Can you work these out from the drawing? Everything is in mm from the part's minimum corner. A direction names the side the tool comes from. Give positions to 0.01 mm unless a question says otherwise; leave off trailing zeros. Order: outer loops, then holes, each group sorted by start corner. A loop starts at its lowest first (then second) coordinate and runs counter-clockwise, first axis right, second up. Notation, with made-up numbers: M 60.5,67 L 77.5,67 A21 cw 77.5,101 Z; hole C -21.5,80 d1. An arc over 180 degrees is marked long. Use a Markdown table: item, result. Add a question column.
Item 1: If I drill on L1, parallel to X at y = 9, z = 31; L2, parallel to X at y = 4, z = 8; L3, parallel to Y at x = 5, z = 28.5, over which ranges is the centre line in solid material (lowest first)? Write a range as from..to.
Item 2: For the marked faces 4 and 5, which set-ups out of +Z, -Z, +X, -X, +Y, -Y let a thin tool reach every point of the face, with its end or its side?
Item 3: If we mould it in two halves opening along X, with no side actions, what happens to the marked faces 1, 2 and 3? For each: released by +X, released by -X, zero draft, split by the parting line, or undercut.
Item 4: Suppose I cut it at A-A on z = 44.5. Write out the boundary of the cut face in (x, y).
Item 5: I'm going to push a flat-ended pin straight in: pin 1 Ø3.5 at (x, z) = (4.5, 47) entering from -Y. Where does the tip first touch, or does it pass through?
Item 6: Suppose I cut it at B-B on y = 2.25. Write out the boundary of the cut face in (x, z).
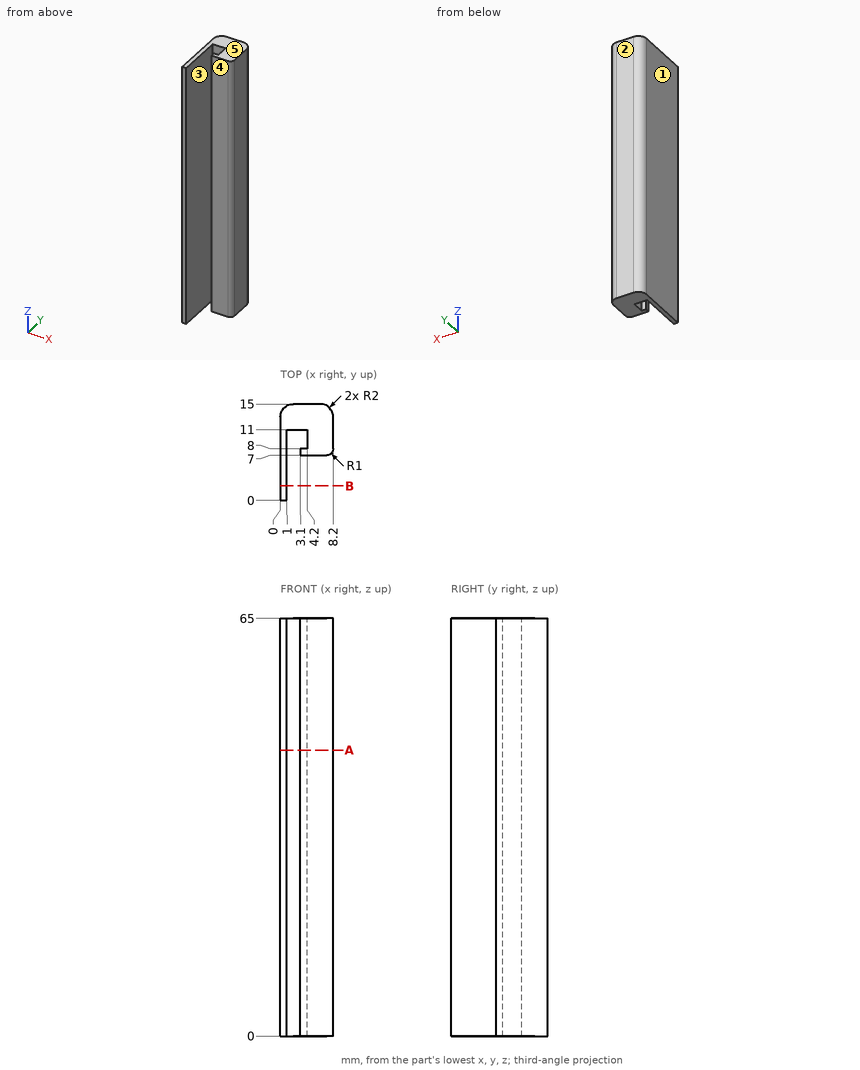
Findings below:
| question | item | result |
|---|---|---|
| 1 | L1 | x = 0..1, 4.2..8.2 |
| 1 | L2 | x = 0..1 |
| 1 | L3 | y = 7..15 |
| 2 | face 4 | +Z, -Z, +X, -Y |
| 2 | face 5 | +Z, +X, -X, +Y, -Y |
| 3 | face 1 | released by -X |
| 3 | face 2 | zero draft |
| 3 | face 3 | undercut |
| 4 | outline | M 0,0 L 1,0 L 1,11 L 4.2,11 L 4.2,8 L 3.1,8 L 3.1,7 L 7.2,7 A1 ccw 8.2,8 L 8.2,13 A2 ccw 6.2,15 L 2,15 A2 ccw 0,13 Z |
| 5 | pin 1 | stops at y = 7 |
| 6 | outline | M 0,0 L 1,0 L 1,65 L 0,65 Z |
